from build123d import *

# Parameters (mm, degrees)
F0_R      = 27
F1_DEPTH  = 45
F2_R      = 41.8433440982
F2_R_2    = 20
F3_DEPTH  = 11
F5_D      = 6.5
F5_DEPTH  = 50
F5_TIP    = 1.9527970118
F6_R      = 5.25
F7_DEPTH  = 40
F8_R      = 2.9
F9_DEPTH  = 3.8
F10_R     = 2.4
F11_DEPTH = 8
F12_R     = 6
F12_R_2   = 3.2524774455
F13_DEPTH = 1
F15_DEPTH = 12
F16_R     = 45.2689658455
F16_R_2   = 30
F17_DEPTH = 53.4


# Not quite as in the source:
# - a feature names something its author has since deleted; it is built from what else it names


with BuildPart() as f1:
    # F0 (on Front) → F1 (new body)
    with BuildSketch(Plane.XZ):
        Circle(F0_R)
    extrude(amount=F1_DEPTH)

    # F2 (on face) → F3 (cut)
    with BuildSketch(Plane.XZ.offset(45)):
        Circle(F2_R)
        Circle(F2_R_2, mode=Mode.SUBTRACT)
    extrude(amount=-F3_DEPTH, mode=Mode.SUBTRACT)

    # F5
    with Locations(Plane(origin=(0, 0, 0), x_dir=(-1, 0, 0), z_dir=(0, 1, 0))):
        with Locations((-9.8994949366, 9.8994949366), (9.8994949366, 9.8994949366), (-9.8994949366, -9.8994949366)):
            Hole(F5_D / 2, depth=F5_DEPTH)
            with Locations((0, 0, -(F5_DEPTH + F5_TIP / 2))):  # 118° drill point
                Cone(0, F5_D / 2, F5_TIP, mode=Mode.SUBTRACT)

    # F6 (on face) → F7 (cut)
    with BuildSketch(Plane(origin=(0, 0, 0), x_dir=(-1, 0, 0), z_dir=(0, 1, 0))):
        with Locations((-9.8994949366, -9.8994949366)):
            Circle(F6_R)
        with Locations((9.8994949366, 9.8994949366)):
            Circle(F6_R)
        with Locations((-9.8994949366, 9.8994949366)):
            Circle(F6_R)
    extrude(amount=-F7_DEPTH, mode=Mode.SUBTRACT)

    # F8 (on face) → F9 (join)
    with BuildSketch(Plane.XZ.offset(45)):
        Circle(F8_R)
    extrude(amount=F9_DEPTH)

    # F10 (on face) → F11 (cut)
    with BuildSketch(Plane.XZ.offset(48.8)):
        Circle(F10_R)
    extrude(amount=-F11_DEPTH, mode=Mode.SUBTRACT)

    # F12 (on face) → F13 (cut)
    with BuildSketch(Plane.XZ.offset(45)):
        Circle(F12_R)
        Circle(F12_R_2, mode=Mode.SUBTRACT)
    extrude(amount=-F13_DEPTH, mode=Mode.SUBTRACT)

    # F14 (on face) → F15 (cut)
    with BuildSketch(Plane(origin=(0, 0, 0), x_dir=(-1, 0, 0), z_dir=(0, 1, 0))):
        Polygon((39.7908514319, 0), (0, 0), (-37.339406552, 0), (-37.339406552, -12), (41.6823292512, -12), align=None)
    extrude(amount=-F15_DEPTH, mode=Mode.SUBTRACT)

    # F16 (on face) → F17 (cut)
    with BuildSketch(Plane(origin=(0, 0, 0), x_dir=(-1, 0, 0), z_dir=(0, 1, 0))):
        with Locations((-10, 0)):
            Circle(F16_R)
        with Locations((-10, 0)):
            Circle(F16_R_2, mode=Mode.SUBTRACT)
    extrude(amount=-F17_DEPTH, mode=Mode.SUBTRACT)


solid = f1.part
Geometry: final body of the model. Coordinates: model frame, mm. A direction names the side the tool comes from. Give positions to 0.01 mm unless a question says otherwise; leave off trailing zeros. Write each loop counter-clockwise with the first axis right and the second up, starting at its lowest first coordinate (ties: lowest second). Pieces come first, ordered by that corner, then holes. Notation, with made-up numbers: (10, -5.5) -> (60, -5.5) arc R37 cw to (60, 32.5) -> close; hole circle Ø11 at (17.25, 62.5). An arc over 180 degrees is marked (long way). Answer in a Markdown table with one row per item.
(1) Set-up query: faces 5 (the flat face through (20, -6, -12)), 6 (the flat face through (3, 0, -18)), 7 (the cylindrical face through (11.038, -24.164, -15.025)), 8 (the flat face through (0, -40.8, 0)). Return all of +Z, -Z, +X, -X, +Y, -Y with unobstructed straight access to the full face (end or side cutting, diameter ignored); none if empty.
Answers below:
| item | result |
|---|---|
| face 5 | +X, -X, +Y |
| face 6 | +Z, -Z, +X, -X, +Y |
| face 7 | +Y |
| face 8 | -Y |
(2) Section query A-A on y = -3.5. Return loops of the section in (x, z).
Answers below:
| item | result |
|---|---|
| outline | (-20, 0) -> (27, 0) arc R27 ccw to (-3.55, 26.77) arc R30 ccw to start; (-17.5, -12) arc R30 ccw to (-3.55, -26.77) arc R27 ccw to (24.19, -12) -> (14.71, -12) arc R5.25 cw to (5.09, -12) -> close; hole circle Ø10.5 at (-9.9, 9.9); hole circle Ø10.5 at (9.9, 9.9) |
(3) Section query D-D on y = -13.5. Return loops of the section in (x, z).
Answers below:
| item | result |
|---|---|
| outline | (-3.55, -26.77) arc R27 ccw (long way) to (-3.55, 26.77) arc R30 ccw to start; hole circle Ø10.5 at (-9.9, 9.9); hole circle Ø10.5 at (9.9, -9.9); hole circle Ø10.5 at (9.9, 9.9) |
(4) Section query B-B on x = 0. Return loops of the section in (y, z).
Answers below:
| item | result |
|---|---|
| outline | (-48.8, -2.9) -> (-45, -2.9) -> (-45, -3.25) -> (-44, -3.25) -> (-44, -6) -> (-45, -6) -> (-45, -20) -> (-34, -20) -> (-34, -27) -> (0, -27) -> (0, -12) -> (-12, -12) -> (-12, 0) -> (0, 0) -> (0, 27) -> (-34, 27) -> (-34, 20) -> (-45, 20) -> (-45, 6) -> (-44, 6) -> (-44, 3.25) -> (-45, 3.25) -> (-45, 2.9) -> (-48.8, 2.9) -> (-48.8, 2.4) -> (-40.8, 2.4) -> (-40.8, -2.4) -> (-48.8, -2.4) -> close |
(5) Pin query (flat end, axial travel): pin 1 (3 mm diameter, centred on x = -6.5, y = -31, fed in from +Z); pin 2 (8.5 mm diameter, centred on x = 9.9, z = -9.9, fed in from -Y); pin 3 (6 mm diameter, centred on x = -2.5, y = -9, fed in from +Z); pin 4 (1 mm diameter, centred on y = -10.5, z = -8, fed in from +X). Return the tip coordinate at first contact, or that it passes through.
Answers below:
| item | result |
|---|---|
| pin 1 | z = 25.98 |
| pin 2 | y = -45 |
| pin 3 | z = 27 |
| pin 4 | through |
(6) Section query C-C on z = 17. Return loops of the section in (x, y).
Answers below:
| item | result |
|---|---|
| outline | (-14.72, -34) -> (-10.54, -34) -> (-10.54, -45) -> (10.54, -45) -> (10.54, -34) -> (20.98, -34) -> (20.98, 0) -> (-14.72, 0) -> close |
(7) Ray query, line 1 along Z through (x, y) = (6.5, -10.5); line 2 along Z through (x, y) = (9.5, -31.5); line 3 along Z through (x, y) = (-0.5, -8). Return the intervals inside material, ascending. Write a range as [from, to].
Answers below:
| item | result |
|---|---|
| line 1 | [-26.21, -13.9], [0, 5.9], [13.9, 26.21] |
| line 2 | [-25.27, -15.13], [-4.66, 4.66], [15.13, 25.27] |
| line 3 | [-27, -12], [0, 27] |
(8) Draft query along Z for faces 1 (the cylindrical face through (-0.705, -44.507, -3.175)), 2 (the flat face through (3, 0, 11)), 3 (the cylindrical face through (7.504, -42.535, -7.703)), 4 (the cylindrical face through (-20, -17, 0)). Return one class per face: +Z half, -Z half, draft (parallel to the pull), parting line (faces both ways), or undercut.
Answers below:
| item | result |
|---|---|
| face 1 | undercut |
| face 2 | draft |
| face 3 | undercut |
| face 4 | parting line |
